Model file for the job. Use its own axes, mm. A direction names the side the tool comes from. Round coordinates to 2 decimals unless told otherwise and drop trailing zeros. Order: outer loops, then holes, each group sorted by start corner. A loop starts at its lowest first (then second) coordinate and runs counter-clockwise, first axis right, second up. Notation, with made-up numbers: (17, 12.25) -> (31, 12.25) arc R32 cw to (31, 49.25) -> close; hole circle Ø7 at (73.25, 60). An arc over 180 degrees is marked (long way). Put each result on its own line as item: value. Start each with the question number.
Q1. Flat gauge pins, fed straight in: P1, Ø1, axis at y = 41, z = -3.5, coming from the +X side; P2, Ø3, axis at x = 4, y = 13.5, coming from the +Z side; P3, Ø1.8, axis at x = 0, z = 0, coming from the +Y side. Where does each tip first touch, or does it go through?
Q2. Pull direction Z, two halves, no side cores. Call faces 4 (the face through (-1.74, 44.52, 0.99)), 5 (the face through (-3, 41, -3)), 6 (the face through (-1.724, 44.521, -1.014)), 7 (the face through (-0.9, 4.44, -2.86)): released by +Z, released by -Z, zero draft, split by the parting line, or undercut.
Q3. Probe L1, parallel to Y at x = -1.75, z = -2; L2, parallel to Y at x = 3.5, z = 5; L3, parallel to Y at x = 0.5, z = -3.5. List the from-to ranges inside material, lowest first.
Q4. Cut at D-D, the plane x = 5. List the corners of the cut face in (y, z).
Q5. 3-axis set-ups, long thin cutter, end or side, ignore diameter. For faces 1 (the face through (0, 45, 2)), 2 (the face through (3.905, 25.79, 0.867)), 3 (the face through (2, 10, 0)): which of +Z, -Z, +X, -X, +Y, -Y reach the whole face in a straight line?
Q6. Cut at C-C, the plane y = 37. List the corners of the cut face in (x, z), and give its area (3 significant figures).
Q7. Cut at A-A, the plane x = 0. List the corners of the cut face in (y, z).
Q8. Cut at B-B, the plane z = 1.25. List the corners of the cut face in (x, y), and give its area (3 significant figures).
from build123d import *

# Parameters (mm, degrees)
CUT_EXTRUDE_1_DEPTH = 3


with BuildPart() as part:
    # 草图1 → 旋转1 (revolve)
    with BuildSketch(Plane.XY, mode=Mode.PRIVATE) as revolve_1_sk:
        Polygon((0, 46), (6.5, 46), (6.5, 41), (4, 41), (4, 11), (2, 11), (2, 9), (3, 9), (3, 0), (0, 0), align=None)
    revolve(revolve_1_sk.sketch.rotate(Axis((0, 0, 0), (0, 1, 0)), 90), axis=Axis((0, 0, 0), (0, 1, 0)))

    # 草图2 → 切除-拉伸1 (cut)
    with BuildSketch(Plane(origin=(0, 46, 0), x_dir=(1, 0, 0), z_dir=(0, 1, 0))):
        Polygon((1.154700538, 2), (-1.154700538, 2), (-2.309401077, 0), (-1.154700538, -2), (1.154700538, -2), (2.309401077, 0), align=None)
    extrude(amount=-CUT_EXTRUDE_1_DEPTH, mode=Mode.SUBTRACT)


solid = part.part
Ans:
1. P1: stops at x = 5.77
1. P2: stops at z = 3.12
1. P3: stops at y = 43
2. face 4: undercut
2. face 5: zero draft
2. face 6: undercut
2. face 7: split by the parting line
3. L1: y = 0 to 9, 11 to 46
3. L2: y = 41 to 46
3. L3: y = 11 to 46
4. outline: (41, -4.15) -> (46, -4.15) -> (46, 4.15) -> (41, 4.15) -> close
5. face 1: +Y
5. face 2: -Y
5. face 3: none
6. outline: circle Ø8 at (0, 0)
6. area: 50.3 mm^2
7. outline: (0, -3) -> (9, -3) -> (9, -2) -> (11, -2) -> (11, -4) -> (41, -4) -> (41, -6.5) -> (46, -6.5) -> (46, -2) -> (43, -2) -> (43, 2) -> (46, 2) -> (46, 6.5) -> (41, 6.5) -> (41, 4) -> (11, 4) -> (11, 2) -> (9, 2) -> (9, 3) -> (0, 3) -> close
8. outline: (-6.38, 41) -> (-3.8, 41) -> (-3.8, 11) -> (-1.56, 11) -> (-1.56, 9) -> (-2.73, 9) -> (-2.73, 0) -> (2.73, 0) -> (2.73, 9) -> (1.56, 9) -> (1.56, 11) -> (3.8, 11) -> (3.8, 41) -> (6.38, 41) -> (6.38, 46) -> (1.59, 46) -> (1.59, 43) -> (-1.59, 43) -> (-1.59, 46) -> (-6.38, 46) -> close
8. area: 338 mm^2
